```python
from build123d import *

# Parameters (mm, degrees)
ESBO_O1_R                  = 15
RESSALTO_EXTRUS_O1_DEPTH   = 12.5
RESSALTO_EXTRUS_O2_DEPTH   = 8
FILETE1_R                  = 5
ESBO_O3_R                  = 11
CORTE_EXTRUS_O1_DEPTH      = 62.120606846
CORTE_EXTRUS_O2_REACH      = 53.678
CORTE_EXTRUS_O2_END_RADIUS = 11
ESBO_O6_R                  = 3
FURO_ROSCADO_DE_M62_D      = 5
FILETE2_R                  = 1


with BuildPart() as part:
    # Esboço1 → Ressalto-extrusão1 (new, symmetric)
    with BuildSketch(Plane.XY):
        Circle(ESBO_O1_R)
    extrude(amount=RESSALTO_EXTRUS_O1_DEPTH, both=True)

    # Esboço2 → Ressalto-extrusão2 (add)
    with BuildSketch(Plane(origin=(0, 15, 0), x_dir=(1, 0, 0), z_dir=(0, 1, 0))):
        with BuildLine():
            Line((41.21897785, 12.5), (0, 12.5))
            Line((0, 12.5), (0, -12.5))
            Line((0, -12.5), (41.21897785, -12.5))
            ThreePointArc((41.21897785, -12.5), (53.71897785, 0), (41.21897785, 12.5))
        make_face()
    extrude(amount=-RESSALTO_EXTRUS_O2_DEPTH)

    # Filete1
    filete1_edges = [part.edges().sort_by_distance(p)[0] for p in [
        (13.266499161, 7, 0),
    ]]
    fillet(filete1_edges, radius=FILETE1_R)

    # Esboço3 → Corte-extrusão1 (cut, through all)
    with BuildSketch(Plane(origin=(0, 0, -12.5), x_dir=(-1, 0, 0), z_dir=(0, 0, -1))):
        Circle(ESBO_O3_R)
    extrude(amount=-CORTE_EXTRUS_O1_DEPTH, mode=Mode.SUBTRACT)

    # Corte-extrusão2: up to this cylinder (the profile starts outside it)
    corte_extrus_o2_end = Plane(origin=(0, 0, 0), z_dir=(0, 0, -1)) * Cylinder(CORTE_EXTRUS_O2_END_RADIUS, 130.356, mode=Mode.PRIVATE)
    # Esboço6 → Corte-extrusão2 (cut, up to the surface)
    with BuildSketch(Plane(origin=(10.606601718, -10.606601718, 0), x_dir=(0, 0, -1), z_dir=(0.7071067811865464, -0.7071067811865488, 0)), mode=Mode.PRIVATE) as corte_extrus_o2_sk1:
        with Locations(Location((0, 0, 0), (0, 0, 90))):
            Circle(ESBO_O6_R)
    corte_extrus_o2_tool1 = extrude(corte_extrus_o2_sk1.sketch, amount=-CORTE_EXTRUS_O2_REACH, mode=Mode.PRIVATE) - corte_extrus_o2_end
    add(corte_extrus_o2_tool1.solids().sort_by_distance((10.606602, -10.606602, 0))[0], mode=Mode.SUBTRACT)

    # Furo roscado de M62 (through all)
    with Locations(Plane(origin=(0, 15, 0), x_dir=(1, 0, 0), z_dir=(0, 1, 0))):
        with Locations((41.21897785, 0)):
            Hole(FURO_ROSCADO_DE_M62_D / 2)

    # Filete2
    filete2_edges = [part.edges().sort_by_distance(p)[0] for p in [
        (30.559363296, 7, -12.5),
        (53.71897785, 15, 0),
        (20.609488925, 15, -12.5),
        (20.609488925, 15, 12.5),
        (30.559363296, 7, 12.5),
        (16.191649499, 5.354101966, -12.5),
        (16.191649499, 5.354101966, 12.5),
        (-10.062305899, -11.124297731, -12.5),
        (-10.062305899, -11.124297731, 12.5),
        (53.71897785, 7, 0),
    ]]
    fillet(filete2_edges, radius=FILETE2_R)


solid = part.part
```
Source: CAD feature listing. Evaluate the final solid. Frame: model axes, mm. A direction names the side the tool comes from. Give positions to 0.01 mm unless a question says otherwise; leave off trailing zeros. Order: outer loops, then holes, each group sorted by start corner. A loop starts at its lowest first (then second) coordinate and runs counter-clockwise, first axis right, second up. Notation, with made-up numbers: (73, 78.5) -> (113, 78.5) arc R20 ccw to (113, 113.5) -> close; hole circle Ø1 at (16.5, 64). An arc over 180 degrees is marked (long way). Use a Markdown table: item, result.
Q1. Pull-direction query (Y, two-part tool) for faces 3 (the face through (43.717, 10.944, -0.11)), 4 (the face through (16.15, 5.31, 0.16)), 5 (the face through (6.945, -11.184, 0.132)), 6 (the face through (26, 15, 0)); classes: +Y half, -Y half, draft (parallel to the pull), parting line (faces both ways), or undercut.
A:
| item | result |
|---|---|
| face 3 | draft |
| face 4 | undercut |
| face 5 | undercut |
| face 6 | +Y half |
Q2. Section C-C (y = 9). State how many separate pieces and enclosed holes the cut face has, and give its area (3 significant figures).
A:
| item | result |
|---|---|
| separate pieces | 2 |
| enclosed holes | 1 |
| area | 1,240 mm^2 |
Q3. First-contact query: P1, Ø2, axis at y = -7, z = -0.5, coming from the -X side; P2, Ø6, axis at x = 41.22, z = 0, coming from the -Y side; P3, Ø12, axis at y = 9.5, z = 5, coming from the -X side. Flat tips, straight axial feed; report the tip coordinate or a pass-through.
A:
| item | result |
|---|---|
| P1 | x = -13.75 |
| P2 | y = 7 |
| P3 | x = -14.59 |
Q4. Section B-B (z = 0). Return the cut outline in (x, y).
A:
| item | result |
|---|---|
| outline | (0, 15) arc R15 ccw (long way) to (8.27, -12.51) -> (5.36, -9.6) arc R11 cw (long way) to (9.6, -5.36) -> (12.51, -8.27) arc R15 ccw to (14.92, 1.5) arc R5 cw to (19.9, 7) -> (38.72, 7) -> (38.72, 15) -> close; (43.72, 7) -> (52.72, 7) arc R1 ccw to (53.72, 8) -> (53.72, 14) arc R1 ccw to (52.72, 15) -> (43.72, 15) -> close |
Q5. Material intervals for line 1 (Y direction, x = 0, z = -2.5); line 2 (Y direction, x = -8.5, z = -6); line 3 (X direction, y = 1.5, z = -2.5), sorted ascending. Write a range as [from, to].
A:
| item | result |
|---|---|
| line 1 | [-15, -11], [11, 15] |
| line 2 | [-12.36, -6.98], [6.98, 12.36] |
| line 3 | [-14.92, -10.9], [10.9, 14.92] |
Q6. Section A-A (y = 0). Return the cut outline in (x, z).
A:
| item | result |
|---|---|
| outline | (-15, -11.5) arc R1 ccw to (-14, -12.5) -> (-11, -12.5) -> (-11, 12.5) -> (-14, 12.5) arc R1 ccw to (-15, 11.5) -> close; (11, -12.5) -> (14, -12.5) arc R1 ccw to (15, -11.5) -> (15, 11.5) arc R1 ccw to (14, 12.5) -> (11, 12.5) -> close |
Q7. Access query for faces 1 (the face through (12, 5, -12.5)), 2 (the face through (36, 7, 0)). Directions: +Z, -Z, +X, -X, +Y, -Y. A direction counts if a zero-diameter tool reaches every point of the face in a straight line with its end or side. Return the directions, or none.
A:
| item | result |
|---|---|
| face 1 | -Z, +X, -X, +Y, -Y |
| face 2 | +Z, -Z, +X, -Y |
